Work out the finished part from the listing and answer in its coordinate system (mm). A direction names the side the tool comes from. Round coordinates to 2 decimals unless told otherwise and drop trailing zeros. Write each loop counter-clockwise with the first axis right and the second up, starting at its lowest first coordinate (ties: lowest second). Pieces come first, ordered by that corner, then holes. Notation, with made-up numbers: (59, -32) -> (115, -32) arc R27 cw to (115, 4) -> close; hole circle Ø10 at (88.25, -14.75). An arc over 180 degrees is marked (long way). One line per item, written item: value.
```python
from build123d import *

# Parameters (mm, degrees)
SKETCH001_R = 68.61574
PAD_DEPTH   = 18


with BuildPart() as part:
    # Sketch → Revolution (revolve)
    with BuildSketch(Plane.XY):
        with BuildLine():
            Line((0, 0), (68.71, 0))
            Line((68.71, 0), (72.71, 0))
            Line((72.71, 0), (72.71, 4.73))
            Line((72.71, 4.73), (68.96, 4.73))
            Line((68.96, 4.73), (68.96, 22.29))
            ThreePointArc((0, 12.35), (34.827971, 14.905909), (68.96, 22.29))
            Line((0, 12.35), (0, 0))
        make_face()
    revolve(axis=Axis((0, 0, 0), (0, 1, 0)))

    # Sketch001 (on DatumPlane) → Pad (new body)
    with BuildSketch(Plane(origin=(0, 4.358878, 0), x_dir=(-1, 0, 0), z_dir=(0, 1, 0))):
        Circle(SKETCH001_R)
        with BuildLine():
            ThreePointArc((45.123091, 34.867908), (33.518525, 46.134291), (19.217549, 53.689385))
            ThreePointArc((-19.217549, 53.689385), (0, 37.520215), (19.217549, 53.689385))
            ThreePointArc((-19.217549, 53.689385), (-33.518525, 46.134291), (-45.123091, 34.867908))
            ThreePointArc((-57.000189, -1.686043), (-35.683845, 11.594384), (-45.123091, 34.867908))
            ThreePointArc((-57.000189, -1.686043), (-54.234112, -17.621731), (-47.105153, -32.139833))
            ThreePointArc((-16.010505, -54.731417), (-22.053829, -30.354491), (-47.105153, -32.139833))
            ThreePointArc((-16.010505, -54.731417), (0, -57.02512), (16.010505, -54.731417))
            ThreePointArc((47.105153, -32.139833), (22.053829, -30.354491), (16.010505, -54.731417))
            ThreePointArc((47.105153, -32.139833), (54.234112, -17.621731), (57.000189, -1.686043))
            ThreePointArc((45.123091, 34.867908), (35.683845, 11.594384), (57.000189, -1.686043))
        make_face(mode=Mode.SUBTRACT)
    extrude(amount=PAD_DEPTH)


solid = part.part
```
(1) A tool of negligible diameter and unlimited length cuts with its end or side. For faces 1 (the face through (-72.64, 2.4, -3.2)), 2 (the face through (-54.724, 13.633, 41.961)), from which of +Z, -Z, +X, -X, +Y, -Y can it reach the whole face along a straight path? Write none if from no direction.
Reported:
face 1: +Y, -Y
face 2: +Y
(2) Consider probe 1 along Y at (x, z) = (35, 62); probe 2 along X at (y, z) = (18.25, 12); probe 3 along X at (y, z) = (20.5, 6). Determine where each line is inside the solid, lowest interval first.
Reported:
probe 1: y = 0 to 4.73
probe 2: x = -67.91 to -35.56, 35.56 to 67.91
probe 3: x = -68.7 to -38.57, 38.57 to 68.7
(3) Find section A-A on y = 7. Give the vertices of the cut face in (x, z), plus the area to 3 significant figures.
Reported:
outline: circle Ø137.92 at (0, 0)
area: 14,900 mm2
(4) Flat-ended cylindrical pins translate along their axes: pin 1 Ø1 at (y, z) = (3.5, -34) entering from +X; pin 2 Ø5 at (x, z) = (20.5, -23.5) entering from +Y; pin 3 Ø6 at (x, y) = (36, 12.5) entering from +Z. Find the tip coordinate at first contact, or state that the pin passes through.
Reported:
pin 1: stops at x = 64.53
pin 2: stops at y = 14.74
pin 3: stops at z = 60.55
